Verification items for the finished model (mm, model axes). A direction names the side the tool comes from. Give positions to 0.01 mm unless a question says otherwise; leave off trailing zeros. Write each loop counter-clockwise with the first axis right and the second up, starting at its lowest first coordinate (ties: lowest second). Pieces come first, ordered by that corner, then holes. Notation, with made-up numbers: (-25.5, -33) -> (-20.5, -33) arc R25 cw to (-20.5, -13) -> close; hole circle Ø9 at (-17, 14). An arc over 180 degrees is marked (long way). Write item = value, one per line.
from build123d import *

# Parameters (mm, degrees)
SKETCH1_R           = 19.05
BOSS_EXTRUDE1_DEPTH = 11.43
CUT_EXTRUDE1_DEPTH  = 10.16
FILLET1_R           = 5.08
FILLET2_R           = 5.08


with BuildPart() as part:
    # Sketch1 → Boss-Extrude1 (new, symmetric)
    with BuildSketch(Plane(origin=(0, 0, 0), x_dir=(1, 0, 0), z_dir=(0, 1, 0))):
        with BuildLine():
            Line((-101.6, 19.05), (101.6, 19.05))
            ThreePointArc((101.6, 19.05), (172.695567884, 0), (101.6, -19.05))
            Line((101.6, -19.05), (-101.6, -19.05))
            ThreePointArc((-101.6, -19.05), (-172.695567884, 0), (-101.6, 19.05))
        make_face()
        with Locations(Location((-134.595567884, 0, 0), (0, 0, 270))):
            Circle(SKETCH1_R, mode=Mode.SUBTRACT)
        with Locations(Location((134.595567884, 0, 0), (0, 0, 90))):
            Circle(SKETCH1_R, mode=Mode.SUBTRACT)
    extrude(amount=BOSS_EXTRUDE1_DEPTH, both=True)

    # Sketch2 → Cut-Extrude1 (cut)
    with BuildSketch(Plane(origin=(0, 11.43, 0), x_dir=(1, 0, 0), z_dir=(0, 1, 0))):
        with BuildLine():
            Line((-82.77922336, 8.645829995), (82.77922336, 8.645829995))
            ThreePointArc((82.77922336, 8.645829995), (91.425053355, 0), (82.77922336, -8.645829995))
            Line((82.77922336, -8.645829995), (-82.77922336, -8.645829995))
            ThreePointArc((-82.77922336, -8.645829995), (-91.425053355, 0), (-82.77922336, 8.645829995))
        make_face()
    cut_extrude1 = extrude(amount=-CUT_EXTRUDE1_DEPTH, mode=Mode.SUBTRACT)

    # Mirror2: Cut-Extrude1 across plane
    add(cut_extrude1.mirror(Plane.ZX), mode=Mode.SUBTRACT)

    # Fillet1
    fillet1_edges = [part.edges().sort_by_distance(p)[0] for p in [
        (101.6, 0, 19.05),
        (-101.6, 0, 19.05),
        (-101.6, 0, -19.05),
        (101.6, 0, -19.05),
    ]]
    fillet(fillet1_edges, radius=FILLET1_R)

    # Fillet2
    fillet2_edges = [part.edges().sort_by_distance(p)[0] for p in [
        (-172.695567884, -11.43, 0),
        (-172.695567884, 11.43, 0),
        (0, -11.43, -19.05),
        (0, 11.43, -19.05),
        (0, -11.43, 19.05),
        (0, 11.43, 19.05),
        (172.695567884, -11.43, 0),
        (172.695567884, 11.43, 0),
        (-101.172887096, -11.43, -19.645157554),
        (-101.172887096, 11.43, -19.645157554),
        (-101.172887096, -11.43, 19.645157554),
        (-101.172887096, 11.43, 19.645157554),
        (101.172887096, -11.43, 19.645157554),
        (101.172887096, 11.43, 19.645157554),
        (101.172887096, -11.43, -19.645157554),
        (101.172887096, 11.43, -19.645157554),
    ]]
    fillet(fillet2_edges, radius=FILLET2_R)


solid = part.part
Item 1: Mould release check, pull along X, two halves, no side actions. Record for faces 1 (the flat face through (1, 6, 8.646)), 2 (the flat face through (1, -11.43, 10)): +X half, -X half, draft (parallel to the pull), parting line (faces both ways), or undercut.
Response values:
face_1 = undercut
face_2 = draft
Item 2: Sectioned sample at B-B on x = -61. Record the cut outline in (y, z), then the cut area to 3 significant figures.
Response values:
outline = (-11.43, -13.97) arc R5.08 ccw to (-6.35, -19.05) -> (6.35, -19.05) arc R5.08 ccw to (11.43, -13.97) -> (11.43, -8.65) -> (1.27, -8.65) -> (1.27, 8.65) -> (11.43, 8.65) -> (11.43, 13.97) arc R5.08 ccw to (6.35, 19.05) -> (-6.35, 19.05) arc R5.08 ccw to (-11.43, 13.97) -> (-11.43, 8.65) -> (-1.27, 8.65) -> (-1.27, -8.65) -> (-11.43, -8.65) -> close
area = 497 mm^2
Item 3: Material ranges on line 1 (Z direction, x = -70, y = 6); line 2 (X direction, y = 5.75, z = 5); line 3 (Z direction, x = -83, y = 7), recorded low to high.
Response values:
line_1 = -19.05 to -8.65, 8.65 to 19.05
line_2 = -172.37 to -152.98, -116.21 to -89.83, 89.83 to 116.21, 152.98 to 172.37
line_3 = -19.01 to -8.64, 8.64 to 19.01
Item 4: Sectioned sample at A-A on z = 0. Record the cut outline in (x, y).
Response values:
outline = (-172.7, -6.35) arc R5.08 ccw to (-167.62, -11.43) -> (-153.65, -11.43) -> (-153.65, 11.43) -> (-167.62, 11.43) arc R5.08 ccw to (-172.7, 6.35) -> close; (-115.55, -11.43) -> (-91.43, -11.43) -> (-91.43, -1.27) -> (91.43, -1.27) -> (91.43, -11.43) -> (115.55, -11.43) -> (115.55, 11.43) -> (91.43, 11.43) -> (91.43, 1.27) -> (-91.43, 1.27) -> (-91.43, 11.43) -> (-115.55, 11.43) -> close; (153.65, -11.43) -> (167.62, -11.43) arc R5.08 ccw to (172.7, -6.35) -> (172.7, 6.35) arc R5.08 ccw to (167.62, 11.43) -> (153.65, 11.43) -> close
Item 5: Set-up check for faces 3 (the flat face through (1, 0, 19.05)), 4 (the cylindrical face through (91.423, -6.421, -0.19)), 5 (the cylindrical face through (-172.67, 0.09, 1.36)), 6 (the cylindrical face through (91.423, 6.421, -0.19)), 7 (the flat face through (-1, 0, -19.05)): record each of +Z, -Z, +X, -X, +Y, -Y from which the full face is reachable in a straight line by a thin tool's end or side.
Response values:
face_3 = +Z, +Y, -Y
face_4 = -Y
face_5 = +Y, -Y
face_6 = +Y
face_7 = -Z, +Y, -Y
Item 6: Go/stop test with flat-tipped pins: P1, Ø6.5, axis at x = -42, y = 2, coming from the -Z side; P2, Ø4, axis at x = -130, y = 5, coming from the +Z side; P3, Ø5, axis at x = -34, z = 4, coming from the -Y side; P4, Ø19, axis at x = 20, z = 1.5, coming from the +Y side. Record where each tip stops, or that it passes through.
Response values:
P1 = -19.05
P2 = 38.01
P3 = -1.27
P4 = 11.43
